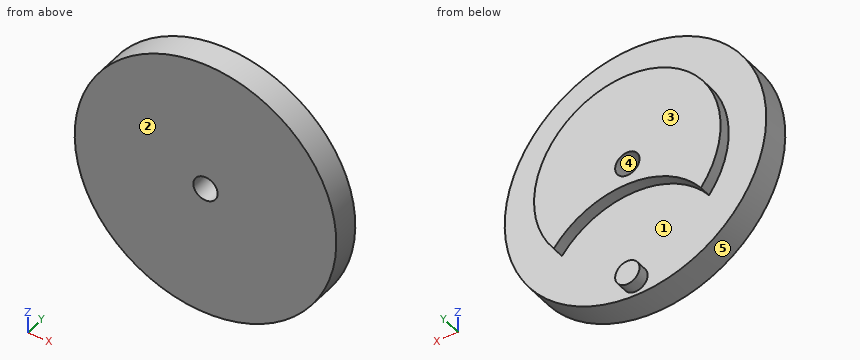
```python
from build123d import *

# Parameters (mm, degrees)
SKETCH1_R           = 64.5
BOSS_EXTRUDE1_DEPTH = 14
SKETCH2_R           = 46
BOSS_EXTRUDE2_DEPTH = 6
SKETCH3_R           = 46
CUT_EXTRUDE3_DEPTH  = 6
SKETCH4_R           = 6
BOSS_EXTRUDE3_DEPTH = 6
SKETCH6_R           = 6
CUT_EXTRUDE2_DEPTH  = 94.383617407


with BuildPart() as part:
    # Sketch1 → Boss-Extrude1 (new body)
    with BuildSketch(Plane(origin=(0, 0, 0), x_dir=(1, 0, 0), z_dir=(0, 1, 0))):
        with Locations(Location((0, 0, 0), (0, 0, 270))):
            Circle(SKETCH1_R)
    extrude(amount=BOSS_EXTRUDE1_DEPTH)

    # Sketch2 → Boss-Extrude2 (add)
    with BuildSketch(Plane(origin=(0, 14, 0), x_dir=(1, 0, 0), z_dir=(0, 1, 0))):
        with Locations(Location((0, 0, 0), (0, 0, 270))):
            Circle(SKETCH2_R)
    extrude(amount=BOSS_EXTRUDE2_DEPTH)

    # Sketch3 → Cut-Extrude3 (cut)
    with BuildSketch(Plane(origin=(0, 20, 0), x_dir=(1, 0, 0), z_dir=(0, 1, 0))):
        with Locations((0, 56.55)):
            Circle(SKETCH3_R)
    extrude(amount=-CUT_EXTRUDE3_DEPTH, mode=Mode.SUBTRACT)

    # Sketch4 → Boss-Extrude3 (add)
    with BuildSketch(Plane(origin=(0, 14, 0), x_dir=(1, 0, 0), z_dir=(0, 1, 0))):
        with Locations(Location((0, 56.55, 0), (0, 0, 270))):
            Circle(SKETCH4_R)
    extrude(amount=BOSS_EXTRUDE3_DEPTH)

    # Sketch6 → Cut-Extrude2 (cut, through all)
    with BuildSketch(Plane(origin=(0, 20, 0), x_dir=(1, 0, 0), z_dir=(0, 1, 0))):
        with Locations(Location((0, 0, 0), (0, 0, 270))):
            Circle(SKETCH6_R)
    extrude(amount=-CUT_EXTRUDE2_DEPTH, mode=Mode.SUBTRACT)


solid = part.part
```
The model under review builds one solid part; all positions refer to its coordinate system, in mm. Face numbers are marked on the shaded views. A direction names the side the tool comes from. Give positions to 0.01 mm unless a question says otherwise; leave off trailing zeros. Write each loop counter-clockwise with the first axis right and the second up, starting at its lowest first coordinate (ties: lowest second). Pieces come first, ordered by that corner, then holes. Notation, with made-up numbers: (76, 62) - (110, 62) arc R22 cw to (110, 86) - close; hole circle Ø5 at (15, -33.75). An arc over 180 degrees is marked (long way). Answer in a Markdown table with one row per item. Add a question column.
1. We need section C-C on y = 18. Write out the cut boundary in (x, z) (3 decimals), then the cut area to 3 significant figures.
2. Insertion check: P1, Ø1, axis at y = 15, z = -25.5, coming from the +X side; P2, Ø1, axis at y = 10.5, z = 13.5, coming from the +X side; P3, Ø4, axis at x = -40, y = 13.5, coming from the +Z side; P4, Ø7, axis at x = 0, z = 0, coming from the -Y side. Each pin has a flat end and moves straight along its axis. Give the tip position at first contact, or say it passes through.
3. We need section A-A on x = 0. Write out the cut boundary in (y, z).
4. We need section B-B on z = 0. Write out the cut boundary in (x, y).
5. We need section D-D on y = 10.25. Write out the cut boundary in (x, z), then the cut area to 3 significant figures.
6. Wall thickness on line 1 along X through (y, z) = (7.25, -0.5); line 2 along X through (y, z) = (15.75, 0); line 3 along Y through (x, z) = (-48.5, -11): over which ranges is each line inside the solid? List them lowest first. Write a range as [from, to].
7. Draft analysis for pull direction X (two halves, no side actions). For the marked faces 3, 4 and 5, state which applies: +X half, -X half, draft (parallel to the pull), parting line (faces both ways), or undercut.
8. Tool access review of the marked faces 1 and 2: name each direction out of +Z, -Z, +X, -X, +Y, -Y from which nothing blocks a thin tool from reaching the whole face with its end or side.
Ans:
| question | item | result |
|---|---|---|
| 1 | outline | (-36.284, -28.275) arc R46 cw to (36.284, -28.275) arc R46 ccw (long way) to start; circle Ø12 at (0, -56.55); hole circle Ø12 at (0, 0) |
| 1 | area | 4,850 mm^2 |
| 2 | P1 | stops at x = 38.61 |
| 2 | P2 | stops at x = 63.18 |
| 2 | P3 | stops at z = 52.12 |
| 2 | P4 | passes through |
| 3 | outline | (0, -64.5) - (14, -64.5) - (14, -62.55) - (20, -62.55) - (20, -50.55) - (14, -50.55) - (14, -10.55) - (20, -10.55) - (20, -6) - (0, -6) - close; (0, 6) - (20, 6) - (20, 46) - (14, 46) - (14, 64.5) - (0, 64.5) - close |
| 4 | outline | (-64.5, 0) - (-6, 0) - (-6, 20) - (-46, 20) - (-46, 14) - (-64.5, 14) - close; (6, 0) - (64.5, 0) - (64.5, 14) - (46, 14) - (46, 20) - (6, 20) - close |
| 5 | outline | circle Ø129 at (0, 0); hole circle Ø12 at (0, 0) |
| 5 | area | 13,000 mm^2 |
| 6 | line 1 | x = [-64.5, -5.98], [5.98, 64.5] |
| 6 | line 2 | x = [-46, -6], [6, 46] |
| 6 | line 3 | y = [0, 14] |
| 7 | face 3 | draft |
| 7 | face 4 | undercut |
| 7 | face 5 | parting line |
| 8 | face 1 | +Y |
| 8 | face 2 | +Z, -Z, +X, -X, -Y |
